Could you check a few things on this model? Use its own coordinates, in mm. A direction names the side the tool comes from. Coordinates: 2 decimals unless noted, no trailing zeros. Loops run counter-clockwise (first coordinate to the right, second up) from the corner with the lowest first, then second, coordinate; pieces in that order, holes last.
1) Imagine slicing it at C-C on y = 49. Please give me the cut outline in (x, z), plus the area to 3 significant figures.
2) If I drill on line 1 along Y through (x, z) = (902.5, 7.5); line 2 along Z through (x, y) = (-97, -48); line 3 along Y through (x, z) = (664.5, -14), over which ranges is the centre line in solid material (lowest first)?
3) For faces 1 (the face through (-477.382, -10, 0.7)), 2 (the face through (410, 280.646, 26)), 3 (the face through (410, -7, 0)), which set-ups out of +Z, -Z, +X, -X, +Y, -Y let a thin tool reach every point of the face, with its end or its side?
4) Will these pins go through, and if not, where does the flat tip stop? P1, Ø1, axis at x = 790.5, y = 54, coming from the -Z side; P2, Ø1, axis at x = 253, y = -188, coming from the +Z side; P3, Ø6, axis at x = 664, z = -29.5, coming from the +Y side.
5) Imagine slicing it at B-B on z = 23. Please give me the cut outline in (x, y), plus the area to 3 significant figures.
6) Imagine slicing it at A-A on x = 744. Please give me the cut outline in (y, z), plus the area to 3 significant figures.
```python
from build123d import *

# Parameters (mm, degrees)
F0_W     = 1800
F0_H     = 585
F1_DEPTH = 1
F0_H_2   = 1
F2_DEPTH = 52
F3_W     = 1800
F3_H     = 1
F4_DEPTH = 44


with BuildPart() as f1:
    # F0 (on Top) → F1 (new body)
    with BuildSketch(Plane.XY):
        with Locations((422.617722, -11.85421)):
            Rectangle(F0_W, F0_H)
    extrude(amount=F1_DEPTH)

    # F0 (on Top) → F2 (join)
    with BuildSketch(Plane.XY):
        with Locations((422.617722, 281.14579)):
            Rectangle(F0_W, F0_H_2)
    extrude(amount=F2_DEPTH)

    # F3 (on face) → F4 (join)
    with BuildSketch(Plane(origin=(0, 0, 0), x_dir=(1, 0, 0), z_dir=(0, 0, -1))):
        with Locations((422.617722, 303.85421)):
            Rectangle(F3_W, F3_H)
    extrude(amount=F4_DEPTH)


solid = f1.part
```
Filled in:
1. outline: (-477.38, 0) - (1322.62, 0) - (1322.62, 1) - (-477.38, 1) - close
1. area: 1,800 mm2
2. line 1: y = 280.65 to 281.65
2. line 2: z = 0 to 1
2. line 3: y = -304.35 to -303.35
3. face 1: +Z, -Z, -X, +Y, -Y
3. face 2: +Z, +X, -X, -Y
3. face 3: -Z, +X, -X, +Y
4. P1: stops at z = 0
4. P2: stops at z = 1
4. P3: stops at y = -303.35
5. outline: (-477.38, 280.65) - (1322.62, 280.65) - (1322.62, 281.65) - (-477.38, 281.65) - close
5. area: 1,800 mm2
6. outline: (-304.35, -44) - (-303.35, -44) - (-303.35, 0) - (281.65, 0) - (281.65, 52) - (280.65, 52) - (280.65, 1) - (-304.35, 1) - close
6. area: 681 mm2
